Autodesk Fusion 360 part; units mm, degrees
sketch "Sketch1" plane through (0, 0, 0) normal (0, 0, 1) x (1, 0, 0)
  circle A0 centre (14.5, 177.5) radius 3.5
  line L0 (7.5, 189.5) -> (118.5, 189.5)
  line L1 (123.5, 184.5) -> (123.5, 7.5)
  line L2 (118.5, 2.5) -> (7.5, 2.5)
  line L3 (2.5, 7.5) -> (2.5, 184.5)
  arc A1 (7.5, 189.5) -> (2.5, 184.5) centre (7.5, 184.5) ccw
  arc A2 (123.5, 184.5) -> (118.5, 189.5) centre (118.5, 184.5) ccw
  arc A3 (2.5, 7.5) -> (7.5, 2.5) centre (7.5, 7.5) ccw
  arc A4 (118.5, 2.5) -> (123.5, 7.5) centre (118.5, 7.5) ccw
  arc A5 (118.5, 5.5) -> (120.5, 7.5) centre (118.5, 7.5) ccw
  line L4 (120.5, 184.5) -> (120.5, 7.5)
  arc A6 (120.5, 184.5) -> (118.5, 186.5) centre (118.5, 184.5) ccw
  line L5 (7.5, 186.5) -> (118.5, 186.5)
  arc A7 (7.5, 186.5) -> (5.5, 184.5) centre (7.5, 184.5) ccw
  line L6 (5.5, 7.5) -> (5.5, 184.5)
  arc A8 (5.5, 7.5) -> (7.5, 5.5) centre (7.5, 7.5) ccw
  line L7 (118.5, 5.5) -> (7.5, 5.5)
  line L8 (63, 186.5) -> (63, 5.5)
  line L9 (5.5, 96) -> (120.5, 96)
  circle A9 centre (111.5, 177.5) radius 3.5
  circle A10 centre (14.5, 14.5) radius 3.5
  circle A11 centre (111.5, 14.5) radius 3.5
  dimension "d5" = 7
  dimension "d28" = 5
  dimension "d30" = 5
  dimension "d32" = 5
  dimension "d34" = 5
  dimension "d36" = 3
  dimension "d37" = 187
  dimension "d38" = 121
  dimension "d41" = 9
  dimension "d42" = 9
extrude "Extrude5" add sketch "Sketch1" along normal blind 2 contours L0 L1 L2 L3 A1 A2 A3 A4 | A5 L4 L7 L8 L9 | L6 A8 L7 L8 L9 | L4 A6 L5 L8 L9 | L5 A7 L6 L8 L9
extrude "Extrude6" add sketch "Sketch1" along normal blind 7 contours L0 L1 L2 L3 A1 A2 A3 A4
sketch "Skizze3" plane through (2.5, 0, 0) normal (-1, 0, 0) x (0, -1, 0)
  line L0 (-184.5, 0) -> (-7.5, 0)
  line L1 (-7.5, 0) -> (-7.5, 7)
  line L2 (-7.5, 7) -> (-184.5, 7)
  line L3 (-184.5, 7) -> (-184.5, 0)
  line L4 (-184.5, 7) -> (-7.5, 0)
  line L5 (-7.5, 7) -> (-184.5, 0)
  line L6 (-85.75, 4.5) -> (-106.25, 4.5)
  line L7 (-106.25, 4.5) -> (-106.25, 2.5)
  line L8 (-106.25, 2.5) -> (-85.75, 2.5)
  line L9 (-85.75, 2.5) -> (-85.75, 4.5)
  line L10 (-85.75, 4.5) -> (-106.25, 2.5) construction
  line L11 (-106.25, 4.5) -> (-85.75, 2.5) construction
  point P0 (-96, 3.5)
  dimension "d43" = 20.5
  dimension "d44" = 2
extrude "Extrusion7" cut sketch "Skizze3" against normal blind 2.5 contours L4 L5 L7 | L4 L5 L7 L8 L9 | L4 L5 L9 | L4 L5 L6 L7 L9
sketch "Skizze4" plane through (0, 189.5, 0) normal (0, 1, 0) x (-1, 0, 0)
  line L0 (-118.5, 0) -> (-7.5, 0)
  line L1 (-7.5, 0) -> (-7.5, 7)
  line L2 (-7.5, 7) -> (-118.5, 7)
  line L3 (-118.5, 7) -> (-118.5, 0)
  line L4 (-118.5, 7) -> (-7.5, 0)
  line L5 (-7.5, 7) -> (-118.5, 0)
  line L6 (-52.75, 4.5) -> (-73.25, 4.5)
  line L7 (-73.25, 4.5) -> (-73.25, 2.5)
  line L8 (-73.25, 2.5) -> (-52.75, 2.5)
  line L9 (-52.75, 2.5) -> (-52.75, 4.5)
  line L10 (-52.75, 4.5) -> (-73.25, 2.5) construction
  line L11 (-73.25, 4.5) -> (-52.75, 2.5) construction
  point P0 (-63, 3.5)
  dimension "d47" = 20.5
  dimension "d48" = 2
extrude "Extrusion8" cut sketch "Skizze4" against normal blind 2.5 contours L4 L5 L7 | L4 L5 L7 L8 L9 | L4 L5 L9 | L4 L5 L6 L7 L9
sketch "Skizze5" plane through (0, 2.5, 0) normal (0, -1, 0) x (1, 0, 0)
  line L0 (7.5, 0) -> (118.5, 0)
  line L1 (118.5, 0) -> (118.5, 7)
  line L2 (118.5, 7) -> (7.5, 7)
  line L3 (7.5, 7) -> (7.5, 0)
  line L4 (118.5, 7) -> (7.5, 0)
  line L5 (7.5, 7) -> (118.5, 0)
  line L6 (73.25, 4.5) -> (52.75, 4.5)
  line L7 (52.75, 4.5) -> (52.75, 2.5)
  line L8 (52.75, 2.5) -> (73.25, 2.5)
  line L9 (73.25, 2.5) -> (73.25, 4.5)
  line L10 (73.25, 4.5) -> (52.75, 2.5) construction
  line L11 (52.75, 4.5) -> (73.25, 2.5) construction
  point P0 (63, 3.5)
  dimension "d51" = 20.5
  dimension "d52" = 2
extrude "Extrusion9" cut sketch "Skizze5" against normal blind 2.5 contours L4 L5 L7 | L4 L5 L7 L8 L9 | L4 L5 L9 | L4 L5 L6 L7 L9
sketch "Skizze6" plane through (123.5, 0, 0) normal (1, 0, 0) x (0, 1, 0)
  line L0 (7.5, 0) -> (184.5, 0)
  line L1 (184.5, 0) -> (184.5, 7)
  line L2 (184.5, 7) -> (7.5, 7)
  line L3 (7.5, 7) -> (7.5, 0)
  line L4 (7.5, 7) -> (184.5, 0)
  line L5 (184.5, 7) -> (7.5, 0)
  line L6 (106.25, 2.5) -> (85.75, 2.5)
  line L7 (85.75, 2.5) -> (85.75, 4.5)
  line L8 (85.75, 4.5) -> (106.25, 4.5)
  line L9 (106.25, 4.5) -> (106.25, 2.5)
  line L10 (106.25, 2.5) -> (85.75, 4.5) construction
  line L11 (85.75, 2.5) -> (106.25, 4.5) construction
  point P0 (96, 3.5)
  point P1 (96, 3.5)
  dimension "d55" = 20.5
  dimension "d56" = 2
  dimension "d59" = 3.5
extrude "Extrusion10" cut sketch "Skizze6" against normal blind 2.5 contours L4 L5 L7 | L4 L5 L6 L7 L9 | L4 L5 L9 | L4 L5 L7 L8 L9
sketch "Cutout USB" plane through (0, 2.5, 0) normal (0, -1, 0) x (1, 0, 0)
  line L0 (52.75, 4.5) -> (73.25, 4.5)
  line L1 (73.25, 4.5) -> (73.25, 2.5)
  line L2 (73.25, 2.5) -> (52.75, 2.5)
  line L3 (52.75, 2.5) -> (52.75, 4.5)
  line L4 (7.5, 0) -> (118.5, 0)
  line L5 (118.5, 0) -> (118.5, 7)
  line L6 (118.5, 7) -> (7.5, 7)
  line L7 (7.5, 7) -> (7.5, 0)
  line L8 (58, 6.25) -> (68, 6.25)
  line L9 (68, 6.25) -> (68, 7)
  line L10 (68, 7) -> (58, 7)
  line L11 (58, 7) -> (58, 6.25)
  dimension "d64" = 10
  dimension "d65" = 0.75
extrude "Extrude11" cut sketch "Cutout USB" against normal blind 190 contours L6 L8 L9 L10 L11
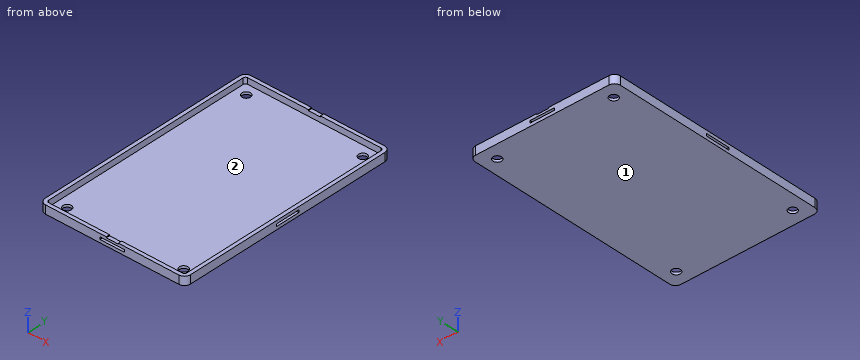
The listing builds one solid part. Answer for the finished solid, in the listing's coordinates (mm). Face numbers are marked on the shaded views. Coordinates: 2 decimals unless noted, no trailing zeros. Order: outer loops, then holes, each group sorted by start corner. A loop starts at its lowest first (then second) coordinate and runs counter-clockwise, first axis right, second up.
Q1. A cutting plane is placed at B-B, the plane y = 14.5. Write down the section's boundary in (x, z), and give its area (3 significant figures).
Q2. A cutting plane is placed at C-C, the plane y = 168. Write down the section's boundary in (x, z).
Q3. Consider line 1 (Y direction, x = 111.5, z = 1.45); line 2 (X direction, y = 177.5, z = 1.1); line 3 (Y direction, x = 18, z = 5). Determine where each line is inside the solid, lowest interval first.
Q4. Given P1, Ø4, axis at x = 14.5, y = 14.5, coming from the +Z side; P2, Ø11, axis at x = 111.5, y = 177.5, coming from the +Z side; P3, Ø1.6, axis at x = 3.5, z = 3.5, coming from the -Y side; P4, Ø0.6, axis at y = 188.5, z = 3.5, coming from the +X side, each flat-ended and moving along its own axis, determine where each tip first touches the part or whether it passes through.
Q5. A cutting plane is placed at A-A, the plane x = 14.5. Write down the section's boundary in (y, z), and give its area (3 significant figures).
Q6. For a pull along Y with two mould halves and no side action, classify the marked faces 1 and 2 as pulls with the +Y half, pulls with the -Y half, needs draft (parallel to the pull), parting line crosses it, or undercut.
Q7. A cutting plane is placed at D-D, the plane x = 98. Write down the section's boundary in (y, z).
Answers follow:
1. outline: (2.5, 0) - (11, 0) - (11, 2) - (5.5, 2) - (5.5, 7) - (2.5, 7) - close; (18, 0) - (108, 0) - (108, 2) - (18, 2) - close; (115, 0) - (123.5, 0) - (123.5, 7) - (120.5, 7) - (120.5, 2) - (115, 2) - close
1. area: 244 mm2
2. outline: (2.5, 0) - (123.5, 0) - (123.5, 7) - (120.5, 7) - (120.5, 2) - (5.5, 2) - (5.5, 7) - (2.5, 7) - close
3. line 1: y = 2.5 to 11, 18 to 174, 181 to 189.5
3. line 2: x = 2.5 to 11, 18 to 108, 115 to 123.5
3. line 3: y = 2.5 to 5.5, 186.5 to 189.5
4. P1: passes through
4. P2: stops at z = 2
4. P3: stops at y = 3.66
4. P4: stops at x = 121.86
5. outline: (2.5, 0) - (11, 0) - (11, 2) - (5.5, 2) - (5.5, 7) - (2.5, 7) - close; (18, 0) - (174, 0) - (174, 2) - (18, 2) - close; (181, 0) - (189.5, 0) - (189.5, 7) - (186.5, 7) - (186.5, 2) - (181, 2) - close
5. area: 376 mm2
6. face 1: needs draft
6. face 2: undercut
7. outline: (2.5, 0) - (189.5, 0) - (189.5, 7) - (186.5, 7) - (186.5, 2) - (5.5, 2) - (5.5, 7) - (2.5, 7) - close
